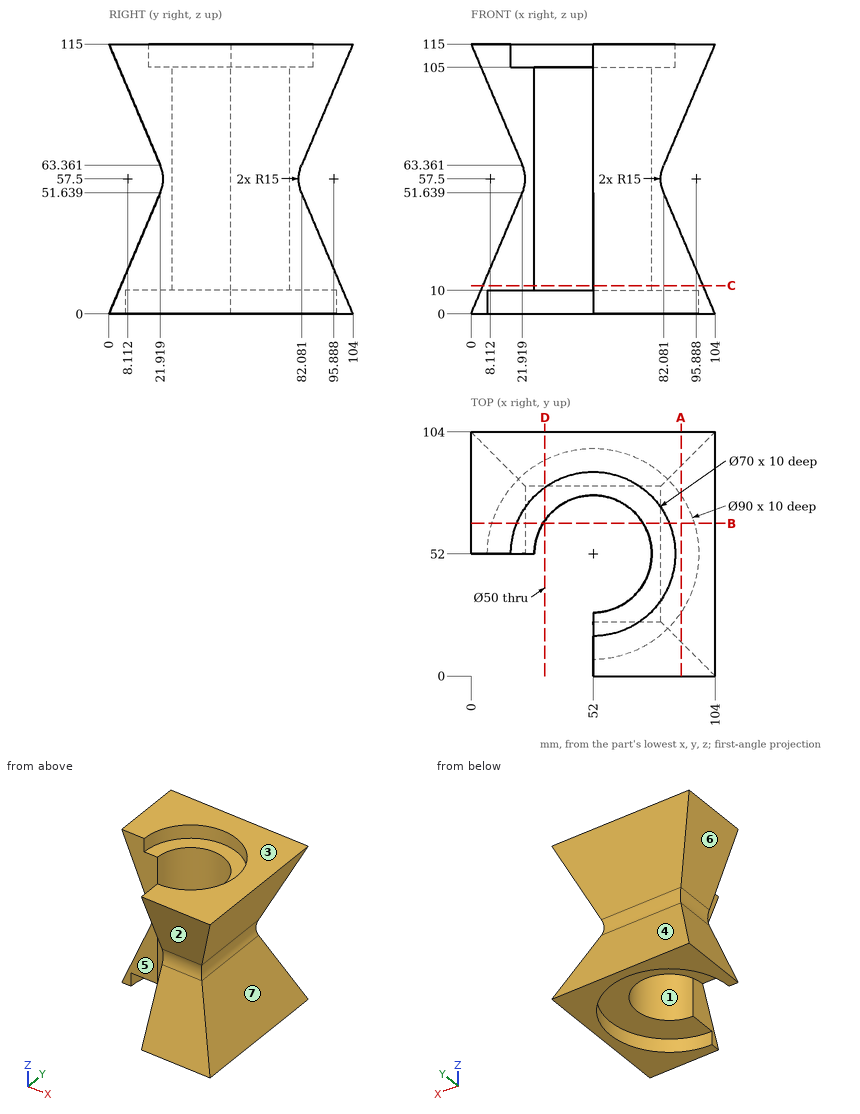
Check sheet for the drawn part. Datum: minimum x, y, z corner. Units: mm. A direction names the side the tool comes from. Give positions to 0.01 mm unless a question says otherwise; leave off trailing zeros. Write each loop counter-clockwise with the first axis right and the second up, starting at its lowest first coordinate (ties: lowest second). Pieces come first, ordered by that corner, then holes. Notation, with made-up numbers: M 77.25,35 L 126.25,35 A34 cw 126.25,74 Z; hole C -32,42 d8. An arc over 180 degrees is marked long. One line per question, with ' | ' between items.
1) Gauge pin test, flat ends, axial feed: pin 1 Ø4 at (x, z) = (18.5, 36.5) entering from +Y (1 decimal); pin 2 Ø21.5 at (y, z) = (12.5, 70) entering from -X; pin 3 Ø5 at (x, z) = (75.5, 62.5) entering from +Y. Record the tip position at first contact, or that the pin passes through.
Result:
pin 1: stops at y = 89.4 | pin 2: stops at x = 52 | pin 3: stops at y = 82.78
2) Section check D-D on x = 31.5. Enter the section's corners in (y, z).
Result:
outline: M 66.31,10 L 92.06,10 L 92.06,0 L 104,0 L 82.08,51.64 A15 cw 82.08,63.36 L 104,115 L 80.37,115 L 80.37,105 L 66.31,105 Z
3) Set-up check for the marked faces 5, 6 and 7: record each of +Z, -Z, +X, -X, +Y, -Y from which the full face is reachable in a straight line by a thin tool's end or side.
Result:
face 5: +Z, -Z, -X, -Y | face 6: -X, +Y, -Y | face 7: +X, +Y, -Y
4) Section check B-B on y = 65. Enter the section's corners in (x, z) (1 decimal).
Result:
outline: M 0,0 L 8.9,0 L 8.9,10 L 30.6,10 L 30.6,105 L 19.5,105 L 19.5,115 L 0,115 L 21.9,63.4 A15 cw 21.9,51.6 Z; M 73.4,10 L 95.1,10 L 95.1,0 L 104,0 L 82.1,51.6 A15 cw 82.1,63.4 L 104,115 L 84.5,115 L 84.5,105 L 73.4,105 Z
5) Mould release check, pull along Z, two halves, no side actions. Record for the marked faces 1, 2, 3 and 4: released by +Z, released by -Z, zero draft, split by the parting line, or undercut.
Result:
face 1: zero draft | face 2: undercut | face 3: released by +Z | face 4: undercut
6) Thickness scan on line 1 along Z through (x, y) = (71.5, 11.5) (1 decimal); line 2 along Z through (x, y) = (96.5, 47) (1 decimal); line 3 along Y through (x, z) = (65, 15) (1 decimal). Record the ranges inside material, lowest first. Write a range as [from, to].
Result:
line 1: z = [10, 27.1], [87.9, 115] | line 2: z = [10, 17.7], [97.3, 115] | line 3: y = [6.4, 30.6], [73.4, 97.6]
7) Section check A-A on x = 89.5. Enter the section's corners in (y, z) (1 decimal).
Result:
outline: M 0,0 L 27.1,0 L 27.1,10 L 76.9,10 L 76.9,0 L 104,0 L 89.5,34.2 L 14.5,34.2 Z; M 0,115 L 14.5,80.8 L 89.5,80.8 L 104,115 Z
8) Section check C-C on z = 12. Enter the section's corners in (x, y).
Result:
outline: M 5.09,52 L 27,52 A25 cw long 52,27 L 52,5.09 L 98.91,5.09 L 98.91,98.91 L 5.09,98.91 Z
